For this review, take the finished solid that the model builds, in its own axes (mm). Face numbers are marked on the shaded views. A direction names the side the tool comes from. Round coordinates to 2 decimals unless told otherwise and drop trailing zeros. Loops run counter-clockwise (first coordinate to the right, second up) from the corner with the lowest first, then second, coordinate; pieces in that order, holes last. Notation, with made-up numbers: (29, 24) -> (39, 24) arc R12 ccw to (39, 41) -> close; hole circle Ø8 at (32, 85). An arc over 180 degrees is marked (long way). One line per question, with ' | ' between items. Start each with the question number.
1. Wall thickness on line 1 along Z through (x, y) = (-6, -16); line 2 along X through (y, z) = (-19.5, 20.5); line 3 along Z through (x, y) = (-26, -5.5): over which ranges is each line inside the solid? List them lowest first.
2. For the marked faces 5 and 6, list the 3-axis set-ups (+Z, -Z, +X, -X, +Y, -Y) from which the entire face can be reached by the end or side of a thin tool; tool diameter is ignored.
3. For pin 1 Ø1.6 at (x, z) = (-6, 5.5) entering from -Y; pin 2 Ø1.6 at (x, z) = (2.5, 25.5) entering from -Y; pin 3 Ø4 at (y, z) = (-14, 14.5) entering from -X; pin 4 Ø4.5 at (y, z) = (-18, 2.5) entering from +X, all flat-tipped, find the tip position at first contact; note any pin that passes through.
4. Consider section D-D (x = -1). Write out the cut boundary in (y, z), and give its area (3 significant figures).
5. Draft analysis for pull direction Z (two halves, no side actions). For the marked faces 1, 2, 3 and 4, state which applies: pulls with the +Z half, pulls with the -Z half, needs draft (parallel to the pull), parting line crosses it, or undercut.
6. Consider section C-C (z = 7.75). Write out the cut boundary in (x, y).
7. Consider section B-B (y = -6). Write out the cut boundary in (x, z).
8. Consider section A-A (y = -23). Write out the cut boundary in (x, z), and give its area (3 significant figures).
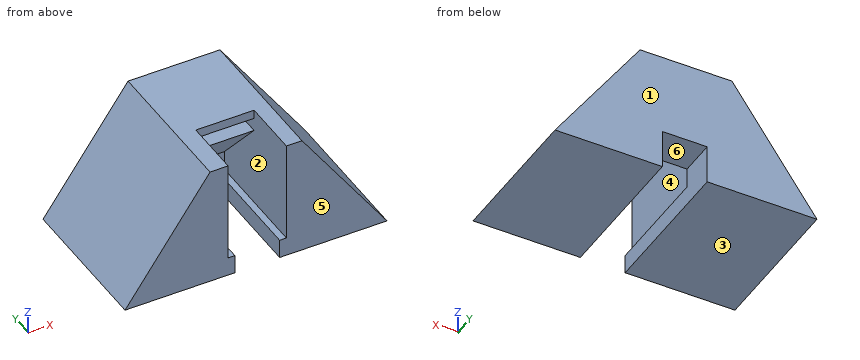
```python
from build123d import *

# Parameters (mm, degrees)
F1_DEPTH = 33
F2_W     = 13
F2_H     = 22.75
F3_DEPTH = 13
F4_W     = 13
F4_H     = 3
F5_DEPTH = 5
F7_DEPTH = 6.5


with BuildPart() as f1:
    # F0 (on Front) → F1 (new body)
    with BuildSketch(Plane.XZ):
        Polygon((-10.527857, 27), (-29.503775, 0), (-5, 0), (-5, 8.67), (5, 8.67), (5, 0), (28.948061, 0), (9.972143, 27), align=None)
    extrude(amount=F1_DEPTH)

    # F2 (on face) → F3 (cut)
    with BuildSketch(Plane.XZ.offset(33)):
        with Locations((0, 15.625)):
            Rectangle(F2_W, F2_H)
    extrude(amount=-F3_DEPTH, mode=Mode.SUBTRACT)

    # F4 (on face) → F5 (cut)
    with BuildSketch(Plane.XZ.offset(20)):
        with Locations((0, 23.5)):
            Rectangle(F4_W, F4_H)
    extrude(amount=-F5_DEPTH, mode=Mode.SUBTRACT)

    # F6 (on Right) → F7 (cut, symmetric)
    with BuildSketch(Plane.YZ):
        Polygon((-8.09, 8.67), (-20, 22), (-20, 4.25), (-8.09, 4.25), align=None)
    extrude(amount=F7_DEPTH, both=True, mode=Mode.SUBTRACT)


solid = f1.part
```
Answer block:
1) line 1: z = 0 to 4.25, 17.52 to 22, 25 to 27 | line 2: x = -15.1 to -6.5, 6.5 to 14.54 | line 3: z = 0 to 4.99
2) face 5: +Z, -Z, +X, -X, -Y | face 6: -Z, +Y, -Y
3) pin 1: stops at y = -33 | pin 2: stops at y = -20 | pin 3: stops at x = -20.72 | pin 4: stops at x = 28.77
4) outline: (-20, 22) -> (-8.09, 8.67) -> (0, 8.67) -> (0, 27) -> (-20, 27) -> (-20, 25) -> (-15, 25) -> (-15, 22) -> close | area: 272 mm2
5) face 1: needs draft | face 2: undercut | face 3: pulls with the -Z half | face 4: undercut
6) outline: (-24.06, -33) -> (-6.5, -33) -> (-6.5, -8.09) -> (-5, -8.09) -> (-5, 0) -> (-24.06, 0) -> close; (5, -8.09) -> (6.5, -8.09) -> (6.5, -33) -> (23.5, -33) -> (23.5, 0) -> (5, 0) -> close
7) outline: (-29.5, 0) -> (-5, 0) -> (-5, 8.67) -> (5, 8.67) -> (5, 0) -> (28.95, 0) -> (9.97, 27) -> (-10.53, 27) -> close
8) outline: (-29.5, 0) -> (-5, 0) -> (-5, 4.25) -> (-6.5, 4.25) -> (-6.5, 27) -> (-10.53, 27) -> close; (5, 0) -> (28.95, 0) -> (9.97, 27) -> (6.5, 27) -> (6.5, 4.25) -> (5, 4.25) -> close | area: 728 mm2
